Check sheet for the modelled part. Datum: model origin and axes. Units: mm. A direction names the side the tool comes from. Round coordinates to 2 decimals unless told otherwise and drop trailing zeros. Loops run counter-clockwise (first coordinate to the right, second up) from the corner with the lowest first, then second, coordinate; pieces in that order, holes last. Notation, with made-up numbers: (26.25, -7) - (32.25, -7) arc R25 cw to (32.25, 7) - close; hole circle Ø6 at (19.5, 72). An arc over 180 degrees is marked (long way). Answer in a Markdown table with one row per item. Add a question column.
(1) Cross-section at B-B on x = 0. Enter the section's corners in (y, z) (1 decimal).
(2) Mould release check, pull along Y, two halves, no side actions. Record for faces 1 (the flat face through (0, -20.32, 0)), 2 (the cylindrical face through (5.037, 14.788, -0.661)), 3 (the flat face through (-1.1, 15.304, 3.3)): +Y half, -Y half, draft (parallel to the pull), parting line (faces both ways), or undercut.
(3) Cross-section at A-A on z = 0. Enter the section's corners in (x, y) (1 decimal).
(4) Cross-section at C-C on y = -8.5. Enter the section's corners in (x, z) (3 decimals).
(5) Cross-section at D-D on x = 4. Enter the section's corners in (y, z), then the cut area to 3 significant figures.
(6) Thickness scan on line 1 along Y through (x, z) = (2.75, -3); line 2 along Y through (x, z) = (-2.75, -1); line 3 along Z through (x, y) = (2, 11.5). Record the ranges inside material, lowest first.
(7) Gauge pin test, flat ends, axial feed: pin 1 (5 mm diameter, centred on x = 0.5, y = 0.5, fed in from -Z) (3 decimals); pin 2 (4 mm diameter, centred on y = 14.5, z = -3.5, fed in from -X); pin 3 (6 mm diameter, centred on y = -0.5, z = -1.5, fed in from +X) (3 decimals). Record the tip position at first contact, or that the pin passes through.
(8) Access from +Z, -Z, +X, -X, +Y, -Y to the whole of each face (thin tool, end or side, straight path). Record for faces 4 (the flat face through (-1.1, 14.288, 3.3)), 5 (the flat face through (0, 22.924, 0)), 6 (the cylindrical face through (-1.93, 18.81, -2.52)).
from build123d import *

# Parameters (mm, degrees)
SKETCH1_R           = 3.175
BOSS_EXTRUDE1_DEPTH = 14.2875
SKETCH3_R           = 5.08
BOSS_EXTRUDE2_DEPTH = 1.016
SKETCH4_R           = 3.175
BOSS_EXTRUDE3_DEPTH = 7.62
CHAMFER2_SIZE       = 0.508
BOSS_EXTRUDE4_START = 20.32
SKETCH9_R           = 3.175
BOSS_EXTRUDE4_DEPTH = 20.32


with BuildPart() as part:
    # Sketch1 → Boss-Extrude1 (new body)
    with BuildSketch(Plane(origin=(0, 0, 0), x_dir=(1, 0, 0), z_dir=(0, 1, 0))):
        with Locations(Location((0, 0, 0), (0, 0, 270))):
            Circle(SKETCH1_R)
    extrude(amount=BOSS_EXTRUDE1_DEPTH)

    # Sketch3 → Boss-Extrude2 (add)
    with BuildSketch(Plane(origin=(0, 14.2875, 0), x_dir=(1, 0, 0), z_dir=(0, 1, 0))):
        with Locations(Location((0, 0, 0), (0, 0, 270))):
            Circle(SKETCH3_R)
    extrude(amount=BOSS_EXTRUDE2_DEPTH)

    # Sketch4 → Boss-Extrude3 (add)
    with BuildSketch(Plane(origin=(0, 15.3035, 0), x_dir=(1, 0, 0), z_dir=(0, 1, 0))):
        with Locations(Location((0, 0, 0), (0, 0, 270))):
            Circle(SKETCH4_R)
    extrude(amount=BOSS_EXTRUDE3_DEPTH)

    # Chamfer2
    chamfer2_edges = [part.edges().sort_by_distance(p)[0] for p in [
        (0, 22.9235, -3.175),
    ]]
    chamfer(chamfer2_edges, length=CHAMFER2_SIZE)

    # Sketch9 → Boss-Extrude4 (add)
    with BuildSketch(Plane.XZ.offset(BOSS_EXTRUDE4_START)):
        with Locations(Location((0, 0, 0), (0, 0, 270))):
            Circle(SKETCH9_R)
    extrude(amount=-BOSS_EXTRUDE4_DEPTH)


solid = part.part
Answers:
| question | item | result |
|---|---|---|
| 1 | outline | (-20.3, -3.2) - (14.3, -3.2) - (14.3, -5.1) - (15.3, -5.1) - (15.3, -3.2) - (22.4, -3.2) - (22.9, -2.7) - (22.9, 2.7) - (22.4, 3.2) - (15.3, 3.2) - (15.3, 5.1) - (14.3, 5.1) - (14.3, 3.2) - (-20.3, 3.2) - close |
| 2 | face 1 | -Y half |
| 2 | face 2 | draft |
| 2 | face 3 | +Y half |
| 3 | outline | (-5.1, 14.3) - (-3.2, 14.3) - (-3.2, -20.3) - (3.2, -20.3) - (3.2, 14.3) - (5.1, 14.3) - (5.1, 15.3) - (3.2, 15.3) - (3.2, 22.4) - (2.7, 22.9) - (-2.7, 22.9) - (-3.2, 22.4) - (-3.2, 15.3) - (-5.1, 15.3) - close |
| 4 | outline | circle Ø6.35 at (0, 0) |
| 5 | outline | (14.29, -3.13) - (15.3, -3.13) - (15.3, 3.13) - (14.29, 3.13) - close |
| 5 | area | 6.36 mm^2 |
| 6 | line 1 | y = 14.29 to 15.3 |
| 6 | line 2 | y = -20.32 to 22.66 |
| 6 | line 3 | z = -2.47 to 2.47 |
| 7 | pin 1 | stops at z = -3.175 |
| 7 | pin 2 | stops at x = -4.85 |
| 7 | pin 3 | stops at x = 3.175 |
| 8 | face 4 | -Y |
| 8 | face 5 | +Z, -Z, +X, -X, +Y |
| 8 | face 6 | +Y |
